```python
from build123d import *

# Parameters (mm, degrees)
SKETCH2_W                  = 20
SKETCH2_H                  = 12.7
CUT_EXTRUDE1_DEPTH         = 1.5
F_8_32_TAPPED_HOLE1_D      = 3.4544
F_8_32_TAPPED_HOLE1_DEPTH  = 10.71
F_8_32_TAPPED_HOLE1_TIP    = 1.037806461
SKETCH7_OUTSIDE_W          = 27.958
SKETCH7_OUTSIDE_H          = 29.458
SKETCH7_OUTSIDE_R          = 6.6
CUT_EXTRUDE2_DEPTH         = 2
F_3_8_0_3750_DOWEL_HOLE2_D = 9.525
CUT_EXTRUDE4_START         = 9
SKETCH11_W                 = 18
SKETCH11_H                 = 20
CUT_EXTRUDE4_DEPTH         = 1
F_1_8_0_1250_DOWEL_HOLE1_D = 3.175
CHAMFER1_SIZE              = 0.5


with BuildPart() as part:
    # Sketch1 → Revolve1 (revolve)
    with BuildSketch(Plane(origin=(0, 0, 0), x_dir=(1, 0, 0), z_dir=(0, 1, 0))):
        Polygon((-16.5, 0), (24, 0), (24, 4), (8.5, 4), (8.5, 9), (-10, 9), (-10, 4), (-16.5, 4), align=None)
    revolve(axis=Axis((-16.5, 0, 0), (1, 0, 0)))

    # Sketch2 → Cut-Extrude1 (cut)
    with BuildSketch(Plane.XY.offset(9)):
        Rectangle(SKETCH2_W, SKETCH2_H)
    extrude(amount=-CUT_EXTRUDE1_DEPTH, mode=Mode.SUBTRACT)

    # #8-32 Tapped Hole1
    with Locations(Plane.ZY.offset(16.5)):
        with Locations((0, 0)):
            Hole(F_8_32_TAPPED_HOLE1_D / 2, depth=F_8_32_TAPPED_HOLE1_DEPTH)
            with Locations((0, 0, -(F_8_32_TAPPED_HOLE1_DEPTH + F_8_32_TAPPED_HOLE1_TIP / 2))):  # 118° drill point
                Cone(0, F_8_32_TAPPED_HOLE1_D / 2, F_8_32_TAPPED_HOLE1_TIP, mode=Mode.SUBTRACT)

    # Sketch7 outside → Cut-Extrude2 (cut)
    with BuildSketch(Plane.ZY.offset(10)):
        with Locations((-0.75, 0)):
            Rectangle(SKETCH7_OUTSIDE_W, SKETCH7_OUTSIDE_H)
        Circle(SKETCH7_OUTSIDE_R, mode=Mode.SUBTRACT)
    extrude(amount=-CUT_EXTRUDE2_DEPTH, mode=Mode.SUBTRACT)

    # 3/8 (0.3750) Dowel Hole2 (through all)
    with Locations(Plane.XY.offset(7.5)):
        with Locations((0, 0)):
            Hole(F_3_8_0_3750_DOWEL_HOLE2_D / 2)

    # Sketch11 → Cut-Extrude4 (cut)
    with BuildSketch(Plane(origin=(0, 0, 0), x_dir=(1, 0, 0), z_dir=(0, 1, 0)).offset(CUT_EXTRUDE4_START)):
        Rectangle(SKETCH11_W, SKETCH11_H)
    cut_extrude4 = extrude(amount=-CUT_EXTRUDE4_DEPTH, mode=Mode.SUBTRACT)

    # 1/8 (0.1250) Dowel Hole1 (through all)
    with Locations(Plane(origin=(0, 8, 0), x_dir=(1, 0, 0), z_dir=(0, 1, 0))):
        with Locations((0, 0)):
            Hole(F_1_8_0_1250_DOWEL_HOLE1_D / 2)

    # Mirror1: Cut-Extrude4 across plane
    add(cut_extrude4.mirror(Plane.ZX), mode=Mode.SUBTRACT)

    # Chamfer1
    chamfer1_edges = [part.edges().sort_by_distance(p)[0] for p in [
        (1.5875, 8, 0),
    ]]
    chamfer(chamfer1_edges, length=CHAMFER1_SIZE)


solid = part.part
```
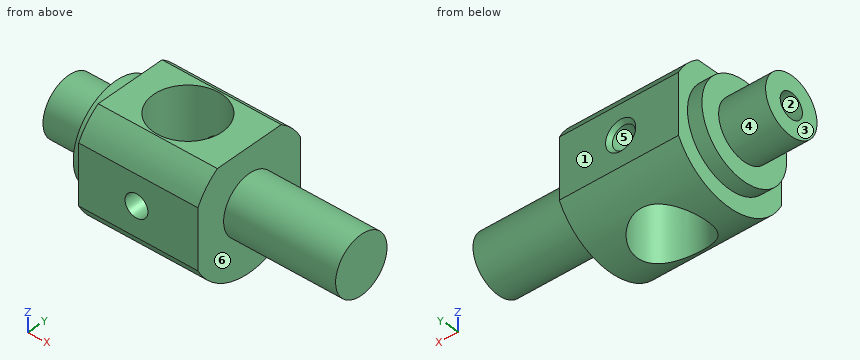
Build history of the part. All positions in model axes, mm. Face numbers are marked on the shaded views. A direction names the side the tool comes from. Round coordinates to 2 decimals unless told otherwise and drop trailing zeros. Loops run counter-clockwise (first coordinate to the right, second up) from the corner with the lowest first, then second, coordinate; pieces in that order, holes last. Notation, with made-up numbers: M 64,-12.75 L 113,-12.75 A13 ccw 113,-2.75 Z; hole C 60.5,-9.75 d10. An arc over 180 degrees is marked long. Answer as CSV lines item,"result".
1. Two-plate mould, pull along Y, no slides. Class the marked faces 1, 2 and 3: released by +Y, released by -Y, zero draft, split by the parting line, or undercut.
Resolved:
face 1,"released by +Y"
face 2,"undercut"
face 3,"zero draft"
2. Cut at A-A on x = -7.5. Write the cut outline in (y, z).
Resolved:
outline,"M -8,-4.12 A9 ccw 8,-4.12 L 8,4.12 A9 ccw 4.97,7.5 L -4.97,7.5 A9 ccw -8,4.12 Z; hole C 0,0 d3.45"
3. Cut at D-D on x = 0. Write the cut outline in (y, z), then the cut area to 3 significant figures.
Resolved:
outline,"M -8,-4.12 A9 ccw -4.76,-7.64 L -4.76,-1.59 L -8,-1.59 Z; M -8,1.59 L -4.76,1.59 L -4.76,7.5 L -4.97,7.5 A9 ccw -8,4.12 Z; M 4.76,-7.64 A9 ccw 8,-4.12 L 8,-2.09 L 7.5,-1.59 L 4.76,-1.59 Z; M 4.76,1.59 L 7.5,1.59 L 8,2.09 L 8,4.12 A9 ccw 4.97,7.5 L 4.76,7.5 Z"
area,"59.4 mm²"
4. Wall check: probe 1 along Y at (x, z) = (0, 3); probe 2 along Y at (x, z) = (13, 0); probe 3 along X at (y, z) = (0, -2). Give the ranges that are in metal, low to high. Write a range as [from, to].
Resolved:
probe 1,"y = [-8, -4.76], [4.76, 8]"
probe 2,"y = [-4, 4]"
probe 3,"x = [-16.5, -4.76], [4.76, 24]"
5. 3-axis set-ups, long thin cutter, end or side, ignore diameter. For the marked faces 4, 5 and 6: which of +Z, -Z, +X, -X, +Y, -Y reach the whole face in a straight line?
Resolved:
face 4,"-X"
face 5,"+Y, -Y"
face 6,"+X"
6. Flat gauge pins, fed straight in: P1, Ø1.5, axis at x = 17.5, z = 0, coming from the +Y side; P2, Ø2, axis at x = 4.5, z = -5.5, coming from the +Y side; P3, Ø2.5, axis at x = 0, z = 0, coming from the -Y side; P4, Ø1, axis at x = 16, z = -3, coming from the +Y side. Where does each tip first touch, or does it go through?
Resolved:
P1,"stops at y = 4"
P2,"stops at y = 7.79"
P3,"passes through"
P4,"stops at y = 3.12"
7. Cut at B-B on y = 2.75. Write the cut outline in (x, z).
Resolved:
outline,"M -16.5,-2.9 L -10,-2.9 L -10,-6 L -8,-6 L -8,-8.57 L -3.89,-8.57 L -3.89,7.5 L -8,7.5 L -8,6 L -10,6 L -10,2.9 L -16.5,2.9 Z; M 3.89,-8.57 L 8.5,-8.57 L 8.5,-2.9 L 24,-2.9 L 24,2.9 L 8.5,2.9 L 8.5,7.5 L 3.89,7.5 Z"
8. Cut at C-C on z = -4.5. Write the cut outline in (x, y) (1 decimal), then the cut area to 3 significant figures.
Resolved:
outline,"M -10,-4.8 L -8,-4.8 L -8,-7.8 L 8.5,-7.8 L 8.5,7.8 L -8,7.8 L -8,4.8 L -10,4.8 Z; hole C 0,0 d9.5"
area,"205 mm²"
